The listing builds one solid part. Answer for the finished solid, in the listing's coordinates (mm). Round coordinates to 2 decimals unless told otherwise and drop trailing zeros. Loops run counter-clockwise (first coordinate to the right, second up) from the corner with the lowest first, then second, coordinate; pieces in that order, holes last. Notation, with made-up numbers: (74, 16) -> (130, 16) arc R7 ccw to (130, 24) -> close; hole circle Ø5 at (44, 6). An arc over 180 degrees is marked (long way). Write each question's results on one line, items separated by ' | '. Start each with the question number.
from build123d import *

# Parameters (mm, degrees)
MODEL_W             = 100
MODEL_H             = 200
MODEL_W_2           = 5.35
MODEL_H_2           = 20
MODEL_W_3           = 11
MODEL_H_3           = 5.35
BOSS_EXTRUDE1_DEPTH = 5.35


with BuildPart() as part:
    # Model → Boss-Extrude1 (new body)
    with BuildSketch(Plane.XY):
        with Locations((50, 100)):
            Rectangle(MODEL_W, MODEL_H)
        with Locations((22.845, 142.5)):
            Rectangle(MODEL_W_2, MODEL_H_2, mode=Mode.SUBTRACT)
        with Locations((77.155, 57.5)):
            Rectangle(MODEL_W_2, MODEL_H_2, mode=Mode.SUBTRACT)
        with Locations((22.845, 100)):
            Rectangle(MODEL_W_2, MODEL_H_2, mode=Mode.SUBTRACT)
        with Locations((22.845, 57.5)):
            Rectangle(MODEL_W_2, MODEL_H_2, mode=Mode.SUBTRACT)
        with Locations((77.155, 100)):
            Rectangle(MODEL_W_2, MODEL_H_2, mode=Mode.SUBTRACT)
        with Locations((77.155, 142.5)):
            Rectangle(MODEL_W_2, MODEL_H_2, mode=Mode.SUBTRACT)
        with Locations((50, 120.75)):
            Rectangle(MODEL_W_3, MODEL_H_3, mode=Mode.SUBTRACT)
        with Locations((50, 79.25)):
            Rectangle(MODEL_W_3, MODEL_H_3, mode=Mode.SUBTRACT)
    extrude(amount=BOSS_EXTRUDE1_DEPTH)


solid = part.part
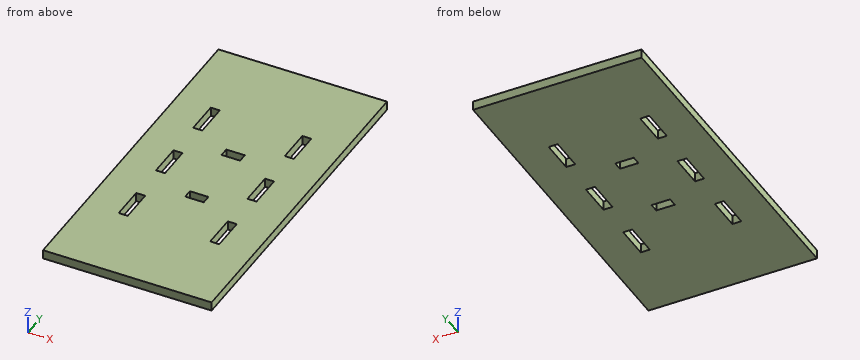
Item 1: The part is cut by section C-C, the plane y = 138.5. Give the vertices of the cut face in (x, z), plus the area to 3 significant figures.
Item 2: Straight lines are drawn through the part: L1, parallel to Y at x = 23.5, z = 3.65; L2, parallel to X at y = 139.5, z = 0.8; L3, parallel to Y at x = 53.5, z = 3.85 (3 decimals). For each, find the intervals that lie inside material, in ascending order. Write a range as [from, to].
Item 3: The part is cut by section D-D, the plane z = 3.7. Give the number of separate pieces and of enclosed holes in the cut face, plus the area to 3 significant figures.
Item 4: The part is cut by section A-A, the plane y = 80. Give the vertices of the cut face in (x, z), plus the area to 3 significant figures.
Item 5: The part is cut by section B-B, the plane x = 50.5. Give the vertices of the cut face in (y, z) (3 decimals), plus the area to 3 significant figures.
Report:
1) outline: (0, 0) -> (20.17, 0) -> (20.17, 5.35) -> (0, 5.35) -> close; (25.52, 0) -> (74.48, 0) -> (74.48, 5.35) -> (25.52, 5.35) -> close; (79.83, 0) -> (100, 0) -> (100, 5.35) -> (79.83, 5.35) -> close | area: 478 mm2
2) L1: y = [0, 47.5], [67.5, 90], [110, 132.5], [152.5, 200] | L2: x = [0, 20.17], [25.52, 74.48], [79.83, 100] | L3: y = [0, 76.575], [81.925, 118.075], [123.425, 200]
3) separate pieces: 1 | enclosed holes: 8 | area: 19,200 mm2
4) outline: (0, 0) -> (44.5, 0) -> (44.5, 5.35) -> (0, 5.35) -> close; (55.5, 0) -> (100, 0) -> (100, 5.35) -> (55.5, 5.35) -> close | area: 476 mm2
5) outline: (0, 0) -> (76.575, 0) -> (76.575, 5.35) -> (0, 5.35) -> close; (81.925, 0) -> (118.075, 0) -> (118.075, 5.35) -> (81.925, 5.35) -> close; (123.425, 0) -> (200, 0) -> (200, 5.35) -> (123.425, 5.35) -> close | area: 1,010 mm2
